Check sheet for the modelled part. Datum: model origin and axes. Units: mm. A direction names the side the tool comes from. Give positions to 0.01 mm unless a question says otherwise; leave off trailing zeros. Loops run counter-clockwise (first coordinate to the right, second up) from the corner with the lowest first, then second, coordinate; pieces in that order, holes last. Notation, with made-up numbers: M -24.75,-38 L 13.25,-38 A36 cw 13.25,1 Z; hole C 15.5,-10.5 d2. An arc over 180 degrees is marked long. Write each question's results on one line, items separated by ' | '. Start each with the question number.
1. Sectioned sample at D-D on z = 8. Record the cut outline in (x, y), and give its area (3 significant figures).
2. Sectioned sample at C-C on x = -4. Record the cut outline in (y, z), and give its area (3 significant figures).
3. Sectioned sample at B-B on y = 11.75. Record the cut outline in (x, z), and give its area (3 significant figures).
4. Sectioned sample at A-A on x = 11. Record the cut outline in (y, z).
5. Go/stop test with flat-tipped pins: pin 1 (1.5 mm diameter, centred on y = 12.5, z = 24.5, fed in from +X); pin 2 (1 mm diameter, centred on y = 12, z = 9, fed in from -X); pin 3 (3.5 mm diameter, centred on x = 11.5, z = 11.5, fed in from +Y); pin 4 (1.6 mm diameter, centred on y = 12, z = 7, fed in from +X). Record where each tip stops, or that it passes through.
6. Tool access check on faces 1 (the flat face through (13, 6.645, 11)), 2 (the flat face through (7.593, 12, 8)), 3 (the flat face through (0, 9.6, -1.7)), 4 (the flat face through (10, 11.176, 4)). Record the directions out of +Z, -Z, +X, -X, +Y, -Y that give a thin tool (end or side, any length) a straight path to the whole face; none if there is none.
7. Material ranges on line 1 along Z through (x, y) = (10, 13.75); line 2 along X through (y, z) = (8, -3); line 3 along Z through (x, y) = (-6, 10), recorded low to high.
8. Draft check along Z on faces 5 (the flat face through (11, 11.176, 12)), 6 (the flat face through (8, 14, -6.005)), 7 (the flat face through (12, 15.24, 9)). Enter one of: pulls with the +Z half, pulls with the -Z half, needs draft (parallel to the pull), parting line crosses it, or undercut.
```python
from build123d import *

# Parameters (mm, degrees)
BOSS_EXTRUDE1_DEPTH     = 15.24
CUT_EXTRUDE1_DEPTH      = 2.54
SKETCH3_W               = 34.486175175
SKETCH3_H               = 6.644984791
CUT_EXTRUDE2_DEPTH      = 34.544
CUT_EXTRUDE2_DEPTH_BACK = 19.812
CUT_EXTRUDE3_DEPTH      = 4.064
SKETCH5_W               = 7.563523275
SKETCH5_H               = 2.007464402
CUT_EXTRUDE4_DEPTH      = 6.604
BOSS_EXTRUDE2_DEPTH     = 2.54


with BuildPart() as part:
    # Sketch1 → Boss-Extrude1 (new body)
    with BuildSketch(Plane(origin=(0, 0, 0), x_dir=(1, 0, 0), z_dir=(0, 1, 0))):
        Polygon((0, 0), (21.138647769, 0), (21.138647769, 6.005297662), (28.985570047, 6.005297662), (25.514226291, -34.486175175), (-12.907838022, 6.005297662), (0, 6.005297662), align=None)
    extrude(amount=BOSS_EXTRUDE1_DEPTH)

    # Sketch2 → Cut-Extrude1 (cut)
    with BuildSketch(Plane(origin=(0, 15.24, 0), x_dir=(1, 0, 0), z_dir=(0, 1, 0))):
        Polygon((21.138647769, 0), (28.470734427, 0), (28.985570047, 6.005297662), (21.138647769, 6.005297662), align=None)
        Polygon((0, 0), (-7.209454713, 0), (-12.907838022, 6.005297662), (0, 6.005297662), align=None)
    extrude(amount=-CUT_EXTRUDE1_DEPTH, mode=Mode.SUBTRACT)

    # Sketch3 → Cut-Extrude2 (cut, two sides)
    with BuildSketch(Plane(origin=(0, 0, 0), x_dir=(0, 0, -1), z_dir=(1, 0, 0))) as cut_extrude2_sk:
        with BuildLine():
            Line((6.005297662, 12.7), (3.002648831, 12.7))
            ThreePointArc((3.002648831, 12.7), (5.001853121, 11.946032476), (6.005297662, 10.05966457))
            Line((6.005297662, 10.05966457), (6.005297662, 12.7))
        make_face()
        with BuildLine():
            ThreePointArc((4.147717946, 9.672492396), (3.443027426, 10.729492855), (2.196307404, 10.485509481))
            Line((2.196307404, 10.485509481), (3.808990258, 8.85947531))
            ThreePointArc((3.808990258, 8.85947531), (4.059649291, 9.2321138), (4.147717946, 9.672492396))
        make_face()
        with BuildLine():
            Line((3.808990258, 8.85947531), (2.196307404, 10.485509481))
            ThreePointArc((2.196307404, 10.485509481), (2.189631745, 8.866150969), (3.808990258, 8.85947531))
        make_face()
        with BuildLine():
            ThreePointArc((5.134576738, 7.522914369), (4.155458111, 6.873057978), (3.002648831, 6.644984791))
            Line((3.002648831, 6.644984791), (6.005297662, 6.644984791))
            Line((6.005297662, 6.644984791), (5.134576738, 7.522914369))
        make_face()
        with BuildLine():
            Line((6.005297662, 6.644984791), (6.005297662, 9.285320221))
            ThreePointArc((6.005297662, 9.285320221), (5.716960561, 8.331480044), (5.134576738, 7.522914369))
            Line((5.134576738, 7.522914369), (6.005297662, 6.644984791))
        make_face()
        Polygon((3.002648831, 6.644984791), (0, 6.644984791), (0, 0), (6.005297662, 0), (6.005297662, 6.644984791), align=None)
        with Locations((-17.243087587, 3.322492396)):
            Rectangle(SKETCH3_W, SKETCH3_H)
    extrude(amount=CUT_EXTRUDE2_DEPTH, mode=Mode.SUBTRACT)
    extrude(cut_extrude2_sk.sketch, amount=-CUT_EXTRUDE2_DEPTH_BACK, mode=Mode.SUBTRACT)

    # Sketch4 → Cut-Extrude3 (cut)
    with BuildSketch(Plane(origin=(0, 15.24, 0), x_dir=(1, 0, 0), z_dir=(0, 1, 0))):
        Polygon((10.569323885, -5.914326858), (10.569323885, -1.709556921), (4.167807975, -1.709556921), (5.834265352, -5.914326858), align=None)
        Polygon((16.948973736, -1.709556921), (10.569323885, -1.709556921), (10.569323885, -5.914326858), (16.077118552, -5.914326858), align=None)
        Polygon((10.569323885, -14.423980302), (10.569323885, -10.352695125), (7.593303694, -10.352695125), (9.206857662, -14.423980302), align=None)
        Polygon((15.156826969, -10.352695125), (10.569323885, -10.352695125), (10.569323885, -14.423980302), (14.312649728, -14.423980302), align=None)
    extrude(amount=-CUT_EXTRUDE3_DEPTH, mode=Mode.SUBTRACT)

    # Sketch5 → Cut-Extrude4 (cut)
    with BuildSketch(Plane.XY.offset(10.352695125)):
        with Locations((11.375065332, 12.228803396)):
            Rectangle(SKETCH5_W, SKETCH5_H)
    extrude(amount=-CUT_EXTRUDE4_DEPTH, mode=Mode.SUBTRACT)

    # Sketch6 → Boss-Extrude2 (add)
    with BuildSketch(Plane(origin=(0, 15.24, 0), x_dir=(1, 0, 0), z_dir=(0, 1, 0))):
        Polygon((28.470734427, 0), (28.985570047, 6.005297662), (-12.907838022, 6.005297662), (-7.209454713, 0), align=None)
    extrude(amount=-BOSS_EXTRUDE2_DEPTH)


solid = part.part
```
Output values:
1) outline: M 0.38,6.64 L 27.78,6.64 L 27.78,15.24 L 0.38,15.24 Z; hole M 7.59,11.23 L 15.16,11.23 L 15.16,13.23 L 7.59,13.23 Z | area: 220 mm2
2) outline: M 6.64,-3 A3.03 ccw 9.29,-6.01 L 10.06,-6.01 A3.03 ccw 12.7,-3 L 12.7,-6.01 L 15.24,-6.01 L 15.24,3.38 L 6.64,3.38 Z; hole C 9.67,-3 d2.29 | area: 72.8 mm2
3) outline: M -12.15,-5.2 L 0,-5.2 L 0,0 L 21.14,0 L 21.14,-5.2 L 28.92,-5.2 L 25.51,34.49 Z; hole M 4.17,1.71 L 16.95,1.71 L 16.08,5.91 L 15.16,5.91 L 15.16,10.35 L 14.31,14.42 L 9.21,14.42 L 7.59,10.35 L 7.59,5.91 L 5.83,5.91 Z | area: 597 mm2
4) outline: M 6.64,0 L 12.7,0 L 12.7,-6.01 L 15.24,-6.01 L 15.24,1.71 L 11.18,1.71 L 11.18,5.91 L 11.23,5.91 L 11.23,10.35 L 11.18,10.35 L 11.18,14.42 L 15.24,14.42 L 15.24,19.19 L 6.64,19.19 Z; M 13.23,5.91 L 15.24,5.91 L 15.24,10.35 L 13.23,10.35 Z
5) pin 1: x = 26.43 | pin 2: x = 0.86 | pin 3: y = 15.24 | pin 4: x = 27.94
6) face 1: +Z, -Z, +X, -X, -Y | face 2: none | face 3: -Z, -Y | face 4: +Y
7) line 1: -6.01 to 1.71, 5.91 to 10.35, 14.42 to 18.14 | line 2: -10.06 to 0, 21.14 to 28.73 | line 3: -6.01 to -4.1, -1.91 to 1.27
8) face 5: undercut | face 6: pulls with the -Z half | face 7: needs draft
